from build123d import *

# Parameters (mm, degrees)
RESSALTO_EXTRUS_O2_DEPTH = 25
ESBO_O6_W                = 60
ESBO_O6_H                = 35
CORTE_EXTRUS_O4_DEPTH    = 25
ESBO_O7_R                = 5.5
CORTE_EXTRUS_O5_DEPTH    = 67
CASCA3_START             = 2
CASCA3_DEPTH             = 21
CORTE_EXTRUS_O7_DEPTH    = 67


# Read off the part's stored shape, not the designer's step: Casca3
with BuildPart() as part:
    # Esboço1 → Ressalto-extrusão2 (new body)
    with BuildSketch(Plane.XY):
        Polygon((-60, 2), (-60, 0), (-60, -35), (-60, -37), (2, -37), (22, -37), (37.696905261, -24.665320756), (37.696905261, -10.334679244), (22, 2), (2, 2), align=None)
    extrude(amount=RESSALTO_EXTRUS_O2_DEPTH)

    # Esboço6 → Corte-extrusão4 (cut)
    with BuildSketch(Plane.XY.offset(25)):
        with Locations((-30, -17.5)):
            Rectangle(ESBO_O6_W, ESBO_O6_H)
    extrude(amount=-CORTE_EXTRUS_O4_DEPTH, mode=Mode.SUBTRACT)

    # Esboço7 → Corte-extrusão5 (cut)
    with BuildSketch(Plane(origin=(0, 2, 0), x_dir=(1, 0, 0), z_dir=(0, 1, 0))):
        with Locations(Location((-35, -12.5, 0), (0, 0, 270))):
            Circle(ESBO_O7_R)
    extrude(amount=-CORTE_EXTRUS_O5_DEPTH, mode=Mode.SUBTRACT)

    # Casca3 outline → Casca3 (cut)
    with BuildSketch(Plane.XY.offset(CASCA3_START)):
        Polygon((0, -35), (21.308212264, -35), (35.696905261, -23.693318211), (35.696905261, -11.306681789), (21.308212264, 0), (0, 0), align=None)
    extrude(amount=CASCA3_DEPTH, mode=Mode.SUBTRACT)

    # Esboço8 → Corte-extrusão7 (cut)
    with BuildSketch(Plane.XY.offset(25)):
        with BuildLine():
            ThreePointArc((13.34845263, -17.5), (18.84845263, -23), (24.34845263, -17.5))
            Line((24.34845263, -17.5), (13.34845263, -17.5))
        make_face()
        with BuildLine():
            Line((13.34845263, -17.5), (24.34845263, -17.5))
            ThreePointArc((24.34845263, -17.5), (18.84845263, -12), (13.34845263, -17.5))
        make_face()
    extrude(amount=-CORTE_EXTRUS_O7_DEPTH, mode=Mode.SUBTRACT)


solid = part.part
Could you check a few things on this model? Use its own coordinates, in mm. A direction names the side the tool comes from. Coordinates: 2 decimals unless noted, no trailing zeros. Order: outer loops, then holes, each group sorted by start corner. A loop starts at its lowest first (then second) coordinate and runs counter-clockwise, first axis right, second up. Notation, with made-up numbers: (-13.75, -19) -> (-7.75, -19) arc R13 ccw to (-7.75, -4) -> close; hole circle Ø4 at (19.25, -0.75). An arc over 180 degrees is marked (long way). One line per item, written item: value. Start each with the question number.
1) Which directions (+Z, -Z, +X, -X, +Y, -Y) give clear straight access to the entire face, cutting with the end or side of a thin tool? Please do faces 1 (the flat face through (37.697, -18, 12)), 2 (the flat face through (0, -18, 24)), 3 (the flat face through (-20, -35, 13)).
2) Imagine slicing it at A-A on x = -14. List the corners of the cut face in (y, z) for me, plus the area to 3 significant figures.
3) Imagine slicing it at D-D on y = -17.5. List the corners of the cut face in (x, z) for me.
4) I'm going to push flat-ended pins straight in: pin 1 (1.5 mm diameter, centred on y = -10, z = 17.5, fed in from -X); pin 2 (5 mm diameter, centred on y = -4, z = 4, fed in from -X); pin 3 (4 mm diameter, centred on y = -9, z = 19, fed in from -X). Where does each tip first touch, or does it pass through?
5) If I drill on L1, parallel to Y at x = -32, z = 17.75; L2, parallel to Z at x = 18.5, y = -34.5; L3, parallel to X at y = -35.5, z = 12.5, over which ranges is the centre line in solid material (lowest first)? Write a range as [from, to].
6) Imagine slicing it at C-C on x = -35. List the corners of the cut face in (y, z) for me.
7) We'd pull the mould along Z, two halves only. Please class faces 4 (the flat face through (10, -17, 25)), 5 (the flat face through (28.402, -29.426, 12.353)), 6 (the flat face through (0, -18, 1)): +Z half, -Z half, draft (parallel to the pull), parting line (faces both ways), or undercut.
8) Imagine slicing it at B-B on z = 12.5. List the corners of the cut face in (x, y) for me, plus the area to 3 significant figures.
Answer list:
1. face 1: +Z, -Z, +X, +Y, -Y
1. face 2: +Z, -Z, -X
1. face 3: -X
2. outline: (-37, 0) -> (-35, 0) -> (-35, 25) -> (-37, 25) -> close; (0, 0) -> (2, 0) -> (2, 25) -> (0, 25) -> close
2. area: 100 mm2
3. outline: (0, 0) -> (13.35, 0) -> (13.35, 2) -> (0, 2) -> close; (0, 23) -> (13.35, 23) -> (13.35, 25) -> (0, 25) -> close; (24.35, 0) -> (37.7, 0) -> (37.7, 25) -> (24.35, 25) -> (24.35, 23) -> (35.7, 23) -> (35.7, 2) -> (24.35, 2) -> close
4. pin 1: stops at x = 33.08
4. pin 2: stops at x = 0
4. pin 3: stops at x = 30.22
5. L1: y = [-37, -35], [0, 2]
5. L2: z = [0, 2], [23, 25]
5. L3: x = [-60, -40.5], [-29.5, 23.91]
6. outline: (-37, 0) -> (-35, 0) -> (-35, 7) -> (-37, 7) -> close; (-37, 18) -> (-35, 18) -> (-35, 25) -> (-37, 25) -> close; (0, 0) -> (2, 0) -> (2, 7) -> (0, 7) -> close; (0, 18) -> (2, 18) -> (2, 25) -> (0, 25) -> close
7. face 4: +Z half
7. face 5: undercut
7. face 6: draft
8. outline: (-60, -37) -> (-40.5, -37) -> (-40.5, -35) -> (-60, -35) -> close; (-60, 0) -> (-40.5, 0) -> (-40.5, 2) -> (-60, 2) -> close; (-29.5, -37) -> (22, -37) -> (37.7, -24.67) -> (37.7, -10.33) -> (22, 2) -> (-29.5, 2) -> (-29.5, 0) -> (21.31, 0) -> (35.7, -11.31) -> (35.7, -23.69) -> (21.31, -35) -> (-29.5, -35) -> close
8. area: 386 mm2
